Check sheet for the modelled part. Datum: model origin and axes. Units: mm. Face numbers are marked on the shaded views. A direction names the side the tool comes from. Give positions to 0.01 mm unless a question says otherwise; leave off trailing zeros. Order: outer loops, then holes, each group sorted by start corner. A loop starts at its lowest first (then second) coordinate and runs counter-clockwise, first axis right, second up. Notation, with made-up numbers: (12, 56) -> (53, 56) arc R17 cw to (53, 85) -> close; hole circle Ø1 at (-10, 24.5). An arc over 180 degrees is marked (long way). Write each question's results on one line, items separated by ' | '.
from build123d import *

# Parameters (mm, degrees)
F0_W     = 5
F0_H     = 1.25
F3_DEPTH = 1
F4_COUNT = 16
F4_ANGLE = 337.5
F7_DEPTH = 2.5


with BuildPart() as f1:
    # F0 (on Front) → F1 (revolve)
    with BuildSketch(Plane.XZ):
        with BuildLine():
            Line((0, 9), (-1, 9))
            Line((-1, 9), (-1.8, 0))
            Line((-1.8, 0), (0, 0))
            Line((0, 0), (0, 4))
            Line((0, 4), (0, 5.25))
            Line((0, 5.25), (0, 8))
            Line((0, 8), (5, 8))
            Line((5, 8), (5, 9))
            ThreePointArc((5, 9), (3, 8.582575695), (1, 9))
            Line((1, 9), (0, 9))
        make_face()
        with Locations((2.5, 4.625)):
            Rectangle(F0_W, F0_H)
    revolve(axis=Axis((5, 0, 0), (1, 0, 0)))

    # F2 (on Right) → F3 (join)
    with BuildSketch(Plane.YZ):
        with BuildLine():
            Line((-0.5, 9.5), (-0.5, 8.25))
            Line((-0.5, 8.25), (0.5, 8.25))
            Line((0.5, 8.25), (0.5, 9.5))
            ThreePointArc((0.5, 9.5), (0.4267766953, 9.6767766953), (0.25, 9.75))
            Line((0.25, 9.75), (-0.25, 9.75))
            ThreePointArc((-0.25, 9.75), (-0.4267766953, 9.6767766953), (-0.5, 9.5))
        make_face()
    f3 = extrude(amount=F3_DEPTH)

    # F4: F3 ×16 about axis
    f4_axis = Axis((-1, 0, 0), (1, 0, 0))
    for i in range(1, F4_COUNT):
        add(f3.rotate(f4_axis, i * F4_ANGLE / (F4_COUNT - 1)))

    # F6 (on offset) → F7 (join)
    with BuildSketch(Plane.YZ.offset(4)):
        with BuildLine():
            Line((-3.2525225542, 2.8314155061), (0, 2.8314155061))
            Line((0, 2.8314155061), (3.46874143, 2.8314155061))
            ThreePointArc((3.46874143, 2.8314155061), (0.1081094379, 4.4914928185), (-3.2525225542, 2.8314155061))
        make_face()
    extrude(amount=-F7_DEPTH)


solid = f1.part
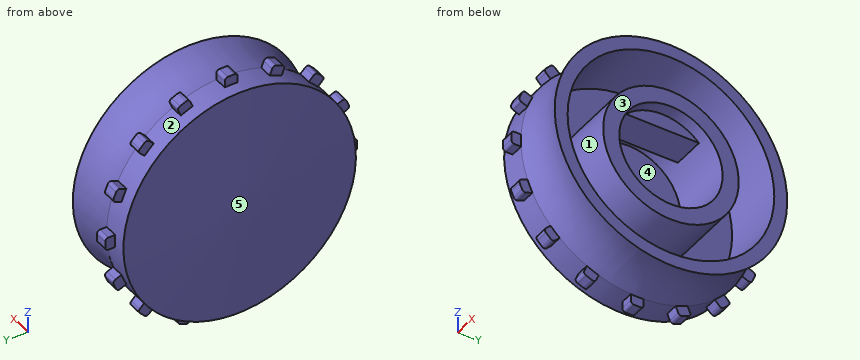
1. Gauge pin test, flat ends, axial feed: pin 1 Ø1.3 at (y, z) = (-6.5, 6.5) entering from -X; pin 2 Ø8 at (y, z) = (-6, 3.5) entering from -X; pin 3 Ø0.6 at (y, z) = (0, 9.5) entering from -X; pin 4 Ø9.5 at (y, z) = (0, 0) entering from +X. Record the tip position at first contact, or that the pin passes through.
Verdict:
pin 1: stops at x = -1.04 | pin 2: stops at x = -1.54 | pin 3: stops at x = 0 | pin 4: stops at x = 5
2. Section check A-A on x = -1.5. Record the cut outline in (y, z) (3 decimals).
Verdict:
outline: circle Ø6.75 at (0, 0)
3. Material ranges on probe 1 along Z at (x, y) = (2.7, 0); probe 2 along Y at (x, z) = (3.6, 0); probe 3 along Y at (x, z) = (1.45, 0), recorded low to high. Write a range as from..to.
Verdict:
probe 1: z = -8.59..-8, -5.25..-4, 2.83..5.25, 8..8.59 | probe 2: y = -8.62..-8, -5.25..-4, 4..5.25, 8..8.62 | probe 3: y = -8.83..-8, -5.25..-4, 4..5.25, 8..8.83
4. Access from +Z, -Z, +X, -X, +Y, -Y to the whole of each face (thin tool, end or side, straight path). Record for the marked faces 1 and 2.
Verdict:
face 1: +X | face 2: -X
5. Mould release check, pull along Y, two halves, no side actions. Record for the marked faces 3, 4 and 5: +Y half, -Y half, draft (parallel to the pull), parting line (faces both ways), or undercut.
Verdict:
face 3: draft | face 4: undercut | face 5: parting line
